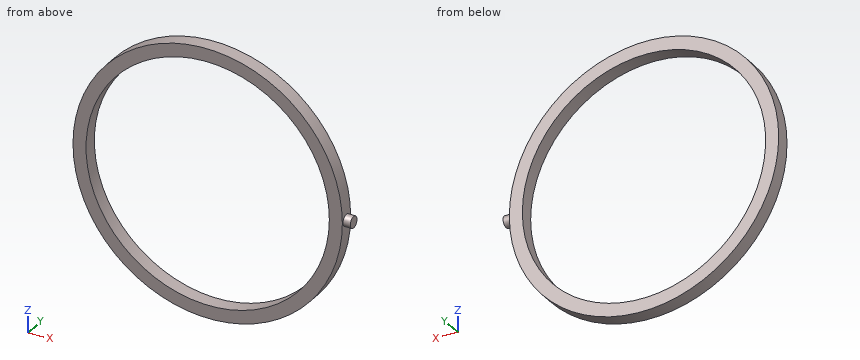
from build123d import *

# Parameters (mm, degrees)
F0_R     = 95
F1_DEPTH = 10
F2_R     = 85.813786
F3_DEPTH = 25
F5_R     = 4.046954
F6_DEPTH = 10


with BuildPart() as f1:
    # F0 (on Front) → F1 (new body)
    with BuildSketch(Plane.XZ):
        Circle(F0_R)
    extrude(amount=F1_DEPTH)

    # F2 (on face) → F3 (cut)
    with BuildSketch(Plane.XZ.offset(10)):
        Circle(F2_R)
    extrude(amount=-F3_DEPTH, mode=Mode.SUBTRACT)

    # F5 (on offset) → F6 (join)
    with BuildSketch(Plane.YZ.offset(90.1)):
        with Locations((-5.129917, 0)):
            Circle(F5_R)
    extrude(amount=F6_DEPTH)


solid = f1.part
Work out the finished part from the listing and answer in its coordinate system (mm). Round coordinates to 2 decimals unless told otherwise and drop trailing zeros. Loops run counter-clockwise (first coordinate to the right, second up) from the corner with the lowest first, then second, coordinate; pieces in that order, holes last. Notation, with made-up numbers: (74.5, 32) - (107.5, 32) arc R18 cw to (107.5, 38) - close; hole circle Ø1 at (55.25, -9). An arc over 180 degrees is marked (long way). One line per item, written item: value.
Q1. Each of these flat-tipped pins is pushed along its axis until it touches: pin 1 Ø6 at (x, y) = (-58.5, -3) entering from -Z; pin 2 Ø2 at (y, z) = (-4.5, 10) entering from -X. Where does it stop, or does it pass through?
Check values:
pin 1: z = -77.1
pin 2: x = -94.57
Q2. Find section D-D on x = -22. Give the vertices of the cut face in (y, z).
Check values:
outline: (-10, -92.42) - (0, -92.42) - (0, -82.95) - (-10, -82.95) - close; (-10, 82.95) - (0, 82.95) - (0, 92.42) - (-10, 92.42) - close
Q3. Straight lines are drawn through the part: probe 1 along Z at (x, y) = (0, -4.25); probe 2 along Z at (x, y) = (77, -7.25); probe 3 along X at (y, z) = (-3.5, 59). For each, find the intervals that lie inside material, in ascending order.
Check values:
probe 1: -95 to -85.81, 85.81 to 95
probe 2: -55.64 to -37.88, 37.88 to 55.64
probe 3: -74.46 to -62.31, 62.31 to 74.46
Q4. Find section A-A on x = 0. Give the vertices of the cut face in (y, z).
Check values:
outline: (-10, -95) - (0, -95) - (0, -85.81) - (-10, -85.81) - close; (-10, 85.81) - (0, 85.81) - (0, 95) - (-10, 95) - close
Q5. Find section B-B on z = 0. Give the vertices of the cut face in (x, y), and give its area (3 significant figures).
Check values:
outline: (-95, -10) - (-85.81, -10) - (-85.81, 0) - (-95, 0) - close; (85.81, -10) - (95, -10) - (95, -9.18) - (100.1, -9.18) - (100.1, -1.08) - (95, -1.08) - (95, 0) - (85.81, 0) - close
area: 225 mm2
Q6. Find section C-C on y = -6.25. Give the vertices of the cut face in (x, z).
Check values:
outline: (94.92, -3.89) - (100.1, -3.89) - (100.1, 3.89) - (94.92, 3.89) arc R95 ccw (long way) to start; hole circle Ø171.63 at (0, 0)
